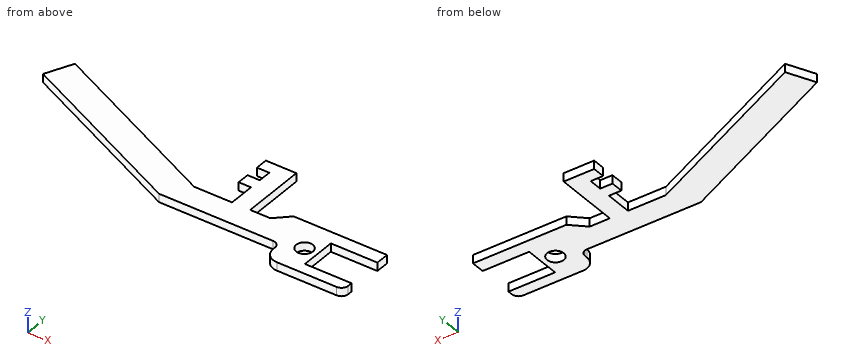
```python
from build123d import *

# Parameters (mm, degrees)
SKETCH1_R           = 1.5875
BOSS_EXTRUDE1_DEPTH = 1.5875


with BuildPart() as part:
    # Sketch1 → Boss-Extrude1 (new body)
    with BuildSketch(Plane.XY):
        with BuildLine():
            Line((-16.325816956, 3.455164033), (-23.558913278, 3.455164033))
            Line((-23.558913278, 3.455164033), (-57.919477855, 19.600489558))
            Line((-57.919477855, 19.600489558), (-60.33041288, 14.469525274))
            Line((-60.33041288, 14.469525274), (-26.855616668, -1.259595838))
            Line((-26.855616668, -1.259595838), (-5.08, -1.259595838))
            ThreePointArc((-5.08, -1.259595838), (-4.181974388, -1.631570226), (-3.81, -2.529595838))
            Line((-3.81, -2.529595838), (-3.81, -3.048))
            ThreePointArc((-3.81, -3.048), (-3.066051224, -4.844051224), (-1.27, -5.588))
            Line((-1.27, -5.588), (10.16, -5.588))
            ThreePointArc((10.16, -5.588), (11.058025612, -5.216025612), (11.43, -4.318))
            Line((11.43, -4.318), (11.43, -3.429))
            Line((11.43, -3.429), (2.54, -3.429))
            Line((2.54, -3.429), (2.54, 3.429))
            Line((2.54, 3.429), (11.43, 3.429))
            Line((11.43, 3.429), (11.43, 5.969))
            Line((11.43, 5.969), (-6.374321652, 5.969))
            Line((-6.374321652, 5.969), (-9.020464775, 3.455164033))
            Line((-9.020464775, 3.455164033), (-12.857372303, 3.455164033))
            Line((-12.857372303, 3.455164033), (-12.857372303, 15.672353851))
            Line((-12.857372303, 15.672353851), (-18.678887174, 15.672353851))
            Line((-18.678887174, 15.672353851), (-18.678887174, 13.324716524))
            Line((-18.678887174, 13.324716524), (-16.325816956, 13.324716524))
            Line((-16.325816956, 13.324716524), (-16.325816956, 10.822176612))
            Line((-16.325816956, 10.822176612), (-18.678887174, 10.822176612))
            Line((-18.678887174, 10.822176612), (-18.678887174, 8.474539284))
            Line((-18.678887174, 8.474539284), (-16.325816956, 8.474539284))
            Line((-16.325816956, 8.474539284), (-16.325816956, 3.455164033))
        make_face()
        Circle(SKETCH1_R, mode=Mode.SUBTRACT)
    extrude(amount=BOSS_EXTRUDE1_DEPTH)


solid = part.part
```
Geometry: final body of the model. Coordinates: model frame, mm. Round coordinates to 2 decimals unless told otherwise and drop trailing zeros. Order: outer loops, then holes, each group sorted by start corner. A loop starts at its lowest first (then second) coordinate and runs counter-clockwise, first axis right, second up. Notation, with made-up numbers: (4, 80) - (37, 80) arc R18 cw to (37, 86) - close; hole circle Ø10 at (-23, 6). An arc over 180 degrees is marked (long way). Write item = value, one per line. Start each with the question number.
Q1. Ray query, line 1 (Y direction, x = 0, z = 1.15); line 2 (X direction, y = 7.75, z = 0.45); line 3 (X direction, y = 7, z = 1.45). Return the intervals inside material, ascending. Write a range as from..to.
Q2. Pin query (flat end, axial travel): pin 1 (0.5 mm diameter, centred on y = 10, z = 0.5, fed in from -X); pin 2 (0.5 mm diameter, centred on x = -11.5, z = 1, fed in from +Y); pin 3 (0.8 mm diameter, centred on x = -17, z = 1, fed in from -Y). Return the tip coordinate at first contact, or that it passes through.
Q3. Cut plane B-B on y = 11.5. Return the cut outline in (x, z).
Q4. Cut plane C-C on z = 0.45. Return the cut outline in (x, y) (1 decimal).
Q5. Cut plane A-A on x = 4. Return the cut outline in (y, z).
Q6. Cut plane D-D on y = 17.5. Return the cut outline in (x, z).
Outcome:
q1.line_1 = -5.59..-1.59, 1.59..5.97
q1.line_2 = -46.03..-32.7, -16.33..-12.86
q1.line_3 = -44.43..-31.1, -16.33..-12.86
q2.pin_1 = -51.35
q2.pin_2 = 3.46
q2.pin_3 = -1.26
q3.outline = (-54.01, 0) - (-40.68, 0) - (-40.68, 1.59) - (-54.01, 1.59) - close; (-16.33, 0) - (-12.86, 0) - (-12.86, 1.59) - (-16.33, 1.59) - close
q4.outline = (-60.3, 14.5) - (-26.9, -1.3) - (-5.1, -1.3) arc R1.3 cw to (-3.8, -2.5) - (-3.8, -3) arc R2.5 ccw to (-1.3, -5.6) - (10.2, -5.6) arc R1.3 ccw to (11.4, -4.3) - (11.4, -3.4) - (2.5, -3.4) - (2.5, 3.4) - (11.4, 3.4) - (11.4, 6) - (-6.4, 6) - (-9, 3.5) - (-12.9, 3.5) - (-12.9, 15.7) - (-18.7, 15.7) - (-18.7, 13.3) - (-16.3, 13.3) - (-16.3, 10.8) - (-18.7, 10.8) - (-18.7, 8.5) - (-16.3, 8.5) - (-16.3, 3.5) - (-23.6, 3.5) - (-57.9, 19.6) - close; hole circle Ø3.2 at (0, 0)
q5.outline = (-5.59, 0) - (-3.43, 0) - (-3.43, 1.59) - (-5.59, 1.59) - close; (3.43, 0) - (5.97, 0) - (5.97, 1.59) - (3.43, 1.59) - close
q6.outline = (-58.91, 0) - (-53.45, 0) - (-53.45, 1.59) - (-58.91, 1.59) - close
